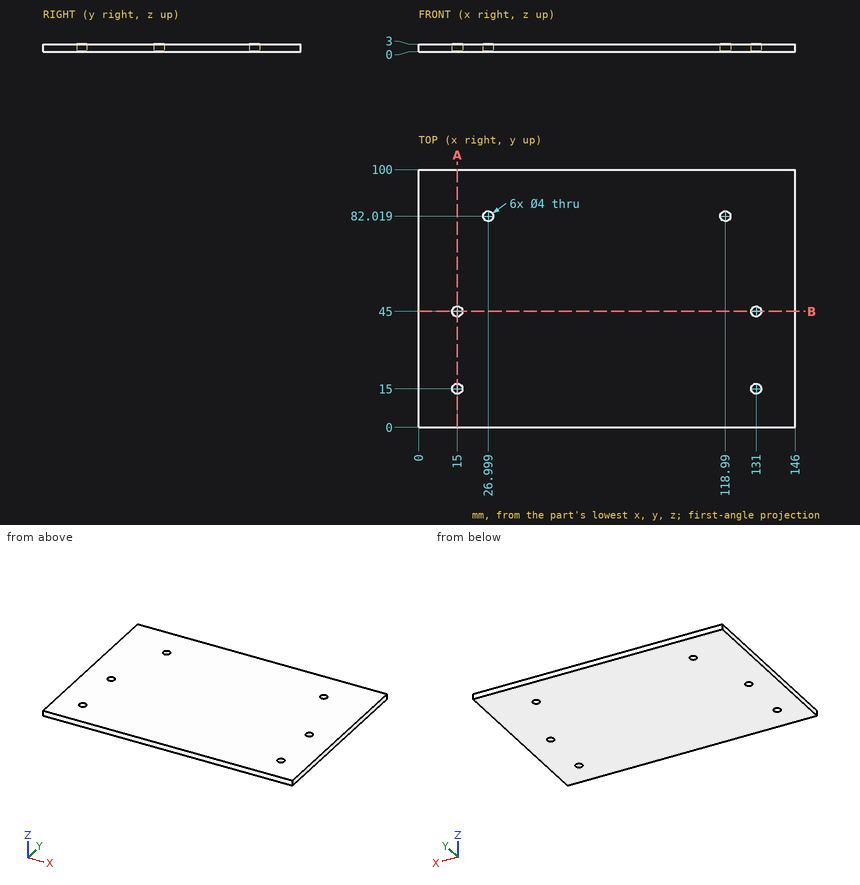
Can you work these out from the drawing? Everything is in mm from the part's minimum corner. Give positions to 0.01 mm unless a question says otherwise; leave off trailing zeros. Order: outer loops, then holes, each group sorted by start corner. A loop starts at its lowest first (then second) coordinate and runs counter-clockwise, first axis right, second up. Notation, with made-up numbers: M -33,84 L -10,84 A25 ccw -10,122 Z; hole C 42.5,40.5 d3. An arc over 180 degrees is marked long. Write item = value, one per line. Start each with the question number.
Q1. Suppose I cut it at B-B (y = 45). Write out the boundary of the cut face in (x, z), plus the area to 3 significant figures.
Q2. I need wall thicknesses on probe 1 along Y at (x, z) = (15, 1.4); probe 2 along X at (y, z) = (82.5, 0.4); probe 3 along Y at (x, z) = (120, 1.65) (1 decimal). Which ranges of each line are inside material? Lowest first, please. Write a range as [from, to].
Q3. Will this pin go through, and if not, where does the flat tip stop? pin 1 Ø2.5 at (x, y) = (118.99, 82.02) entering from +Z.
Q4. Suppose I cut it at A-A (x = 15). Write out the boundary of the cut face in (y, z).
Check result:
q1.outline = M 0,0 L 13,0 L 13,3 L 0,3 Z; M 17,0 L 129,0 L 129,3 L 17,3 Z; M 133,0 L 146,0 L 146,3 L 133,3 Z
q1.area = 414 mm2
q2.probe_1 = [0, 13], [17, 43], [47, 100]
q2.probe_2 = [0, 25.06], [28.94, 117.05], [120.93, 146]
q2.probe_3 = [0, 80.3], [83.7, 100]
q3.pin_1 = through
q4.outline = M 0,0 L 13,0 L 13,3 L 0,3 Z; M 17,0 L 43,0 L 43,3 L 17,3 Z; M 47,0 L 100,0 L 100,3 L 47,3 Z
